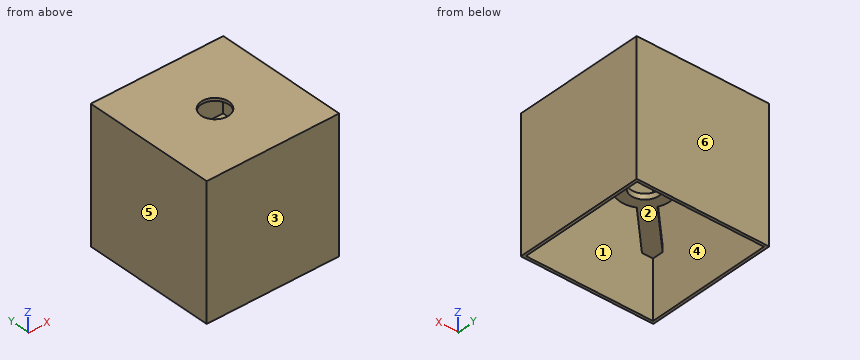
```python
from build123d import *

# Parameters (mm, degrees)
F0_W      = 304.8
F0_H      = 304.8
F0_W_2    = 292.1
F0_H_2    = 292.1
F1_DEPTH  = 152.4
F2_W      = 304.8
F2_H      = 304.8
F3_DEPTH  = 6.35
F5_D      = 0.0254
F5_DEPTH  = 12.7
F6_D      = 0.0254
F6_DEPTH  = 12.7
F8_D      = 0.0254
F8_DEPTH  = 12.7
F9_D      = 0.0254
F9_DEPTH  = 12.7
F12_D     = 0.0254
F12_DEPTH = 12.7
F13_D     = 0.0254
F13_DEPTH = 12.7
F14_D     = 0.0254
F14_DEPTH = 12.7
F15_D     = 0.0254
F15_DEPTH = 12.7
F16_D     = 0.0254
F16_DEPTH = 12.7
F17_D     = 0.0254
F17_DEPTH = 12.7
F19_R     = 31.75
F20_DEPTH = 12.7
F21_R     = 31.75
F22_DEPTH = 25.4


with BuildPart() as f1:
    # F0 (on Top) → F1 (new body, symmetric)
    with BuildSketch(Plane.XY):
        Rectangle(F0_W, F0_H)
        Rectangle(F0_W_2, F0_H_2, mode=Mode.SUBTRACT)
    extrude(amount=F1_DEPTH, both=True)

    # F2 (on face) → F3 (join)
    with BuildSketch(Plane.XY.offset(152.4)):
        Rectangle(F2_W, F2_H)
    extrude(amount=-F3_DEPTH)

    # F5
    with Locations(Plane(origin=(0, 152.4, 0), x_dir=(-1, 0, 0), z_dir=(0, 1, 0))):
        with Locations((38.1, 0)):
            Hole(F5_D / 2, depth=F5_DEPTH)

    # F6
    with Locations(Plane(origin=(0, 152.4, 0), x_dir=(-1, 0, 0), z_dir=(0, 1, 0))):
        with Locations((-106.68, -120.65)):
            Hole(F6_D / 2, depth=F6_DEPTH)

    # F8
    with Locations(Plane.XZ.offset(152.4)):
        with Locations((-106.68, -120.65)):
            Hole(F8_D / 2, depth=F8_DEPTH)

    # F9
    with Locations(Plane.XZ.offset(152.4)):
        with Locations((38.1, 0)):
            Hole(F9_D / 2, depth=F9_DEPTH)

    # F12
    with Locations(Plane.YZ.offset(152.4)):
        with Locations((-114.3, -95.25)):
            Hole(F12_D / 2, depth=F12_DEPTH)

    # F13
    with Locations(Plane.YZ.offset(152.4)):
        with Locations((-120.65, 45.72)):
            Hole(F13_D / 2, depth=F13_DEPTH)

    # F14
    with Locations(Plane(origin=(-152.4, 0, 0), x_dir=(0, -1, 0), z_dir=(-1, 0, 0))):
        with Locations((-114.3, -95.25)):
            Hole(F14_D / 2, depth=F14_DEPTH)

    # F15
    with Locations(Plane(origin=(-152.4, 0, 0), x_dir=(0, -1, 0), z_dir=(-1, 0, 0))):
        with Locations((-120.65, 45.72)):
            Hole(F15_D / 2, depth=F15_DEPTH)

    # F16
    with Locations(Plane(origin=(-152.4, 0, 0), x_dir=(0, -1, 0), z_dir=(-1, 0, 0))):
        with Locations((101.6, 76.2)):
            Hole(F16_D / 2, depth=F16_DEPTH)

    # F17
    with Locations(Plane.YZ.offset(152.4)):
        with Locations((101.6, 76.2)):
            Hole(F17_D / 2, depth=F17_DEPTH)

    # F19 (on offset) → F20 (join)
    with BuildSketch(Plane(origin=(0, 0, -6.35), x_dir=(1, 0, 0), z_dir=(0, 0, -1))):
        with BuildLine():
            Line((120.65, -146.05), (146.05, -146.05))
            Line((146.05, -146.05), (146.05, -120.65))
            Line((146.05, -120.65), (51.063671, -25.663671))
            ThreePointArc((51.063671, -25.663671), (57.15, 0), (51.063671, 25.663671))
            Line((51.063671, 25.663671), (146.05, 120.65))
            Line((146.05, 120.65), (146.05, 146.05))
            Line((146.05, 146.05), (120.65, 146.05))
            Line((120.65, 146.05), (25.663671, 51.063671))
            ThreePointArc((25.663671, 51.063671), (0, 57.15), (-25.663671, 51.063671))
            Line((-25.663671, 51.063671), (-120.65, 146.05))
            Line((-120.65, 146.05), (-146.05, 146.05))
            Line((-146.05, 146.05), (-146.05, 120.65))
            Line((-146.05, 120.65), (-51.063671, 25.663671))
            ThreePointArc((-51.063671, 25.663671), (-57.15, 0), (-51.063671, -25.663671))
            Line((-51.063671, -25.663671), (-146.05, -120.65))
            Line((-146.05, -120.65), (-146.05, -146.05))
            Line((-146.05, -146.05), (-120.65, -146.05))
            Line((-120.65, -146.05), (-25.663671, -51.063671))
            ThreePointArc((-25.663671, -51.063671), (0, -57.15), (25.663671, -51.063671))
            Line((25.663671, -51.063671), (120.65, -146.05))
        make_face()
        Circle(F19_R, mode=Mode.SUBTRACT)
    extrude(amount=F20_DEPTH)

    # F21 (on face) → F22 (cut)
    with BuildSketch(Plane.XY.offset(152.4)):
        Circle(F21_R)
    extrude(amount=-F22_DEPTH, mode=Mode.SUBTRACT)


solid = f1.part
```
Here's how the part is built. I have some questions about the finished solid (model axes, mm). Face numbers are marked on the shaded views. A direction names the side the tool comes from. Give positions to 0.01 mm unless a question says otherwise; leave off trailing zeros. Order: outer loops, then holes, each group sorted by start corner. A loop starts at its lowest first (then second) coordinate and runs counter-clockwise, first axis right, second up. Notation, with made-up numbers: M 25.5,49 L 32.5,49 A34 cw 32.5,86 Z; hole C 34,72.5 d5. An arc over 180 degrees is marked long. Use a Markdown table: item, result. Add a question column.
1. I need wall thicknesses on probe 1 along Y at (x, z) = (118, 3); probe 2 along X at (y, z) = (127, -11.5). Which ranges of each line are inside material? Lowest first, please. Write a range as from..to.
2. If we mould it in two halves opening along X, with no side actions, what happens to the marked faces 4, 5 and 6? For each: +X half, -X half, draft (parallel to the pull), parting line (faces both ways), or undercut.
3. Suppose I cut it at D-D (x = -13.5). List the corners of the cut face in (y, z) for me.
4. On a 3-axis mill with a long thin cutter (end or side, diameter ignored), from which of +Z, -Z, +X, -X, +Y, -Y can I reach the whole of each face in a straight line? I mean the marked faces 1, 2 and 3. Say none if no direction works.
5. For pin 1 Ø4 at (x, y) = (-38.5, 40.5) entering from -Z; pin 2 Ø6 at (x, y) = (78.5, 109) entering from -Z, each with a flat end and sliding along its axis, tell me the tip position at first contact or that it passes through.
6. Suppose I cut it at A-A (y = 66). List the corners of the cut face in (x, z) for me.
7. Suppose I cut it at C-C (y = -37). List the corners of the cut face in (x, z) for me, and give its area (3 significant figures).
8. Suppose I cut it at B-B (z = 69.5). List the corners of the cut face in (x, y) for me.
Results list:
| question | item | result |
|---|---|---|
| 1 | probe 1 | y = -152.4..-146.05, 146.05..152.4 |
| 1 | probe 2 | x = -152.4..-101.6, 101.6..152.4 |
| 2 | face 4 | undercut |
| 2 | face 5 | -X half |
| 2 | face 6 | draft |
| 3 | outline | M -152.4,-152.4 L -146.05,-152.4 L -146.05,146.05 L -28.74,146.05 L -28.74,152.4 L -152.4,152.4 Z; M -55.53,-19.05 L -28.74,-19.05 L -28.74,-6.35 L -55.53,-6.35 Z; M 28.74,-19.05 L 55.53,-19.05 L 55.53,-6.35 L 28.74,-6.35 Z; M 28.74,146.05 L 146.05,146.05 L 146.05,-152.4 L 152.4,-152.4 L 152.4,152.4 L 28.74,152.4 Z |
| 4 | face 1 | none |
| 4 | face 2 | -Z |
| 4 | face 3 | +Z, -Z, +X, -X, -Y |
| 5 | pin 1 | stops at z = -19.05 |
| 5 | pin 2 | stops at z = 146.05 |
| 6 | outline | M -152.4,-152.4 L -146.05,-152.4 L -146.05,146.05 L 146.05,146.05 L 146.05,-152.4 L 152.4,-152.4 L 152.4,152.4 L -152.4,152.4 Z; M -91.4,-19.05 L -40.6,-19.05 L -40.6,-6.35 L -91.4,-6.35 Z; M 40.6,-19.05 L 91.4,-19.05 L 91.4,-6.35 L 40.6,-6.35 Z |
| 7 | outline | M -152.4,-152.4 L -146.05,-152.4 L -146.05,146.05 L 146.05,146.05 L 146.05,-152.4 L 152.4,-152.4 L 152.4,152.4 L -152.4,152.4 Z; M -62.4,-19.05 L 62.4,-19.05 L 62.4,-6.35 L -62.4,-6.35 Z |
| 7 | area | 7,310 mm² |
| 8 | outline | M -152.4,-152.4 L 152.4,-152.4 L 152.4,152.4 L -152.4,152.4 Z; hole M -146.05,-146.05 L 146.05,-146.05 L 146.05,146.05 L -146.05,146.05 Z |
